from build123d import *

# Parameters (mm, degrees)
IZIM1_W                     = 12.4
IZIM1_H                     = 22.6
Y_KSEKLIK_EKSTR_ZYON1_DEPTH = 22.6
Y_KSEKLIK_EKSTR_ZYON2_DEPTH = 2.5
IZIM3_W                     = 3.6
IZIM3_H                     = 3
Y_KSEKLIK_EKSTR_ZYON3_DEPTH = 1.2
IZIM4_R                     = 6.2
Y_KSEKLIK_EKSTR_ZYON4_DEPTH = 4.25
IZIM5_R                     = 2.45
IZIM5_R_2                   = 0.6
Y_KSEKLIK_EKSTR_ZYON6_DEPTH = 3.15
IZIM6_W                     = 0.1
IZIM6_H                     = 1.2
KES_EKSTR_ZYON1_DEPTH       = 3
RADYUS1_R                   = 0.5


with BuildPart() as part:
    # Çizim1 → Yükseklik-Ekstrüzyon1 (new body)
    with BuildSketch(Plane(origin=(0, 0, 0), x_dir=(1, 0, 0), z_dir=(0, 1, 0))):
        Rectangle(IZIM1_W, IZIM1_H)
    extrude(amount=Y_KSEKLIK_EKSTR_ZYON1_DEPTH)

    # Çizim2 → Yükseklik-Ekstrüzyon2 (add)
    with BuildSketch(Plane(origin=(0, 18.2, 0), x_dir=(1, 0, 0), z_dir=(0, 1, 0))):
        with BuildLine():
            Line((-6.2, 16.125), (-6.2, -16.125))
            Line((-6.2, -16.125), (-0.5, -16.125))
            Line((-0.5, -16.125), (-0.5, -15.125))
            ThreePointArc((-0.5, -15.125), (-0.574456265, -13.207120951), (1.1, -14.145204103))
            ThreePointArc((1.1, -14.145204103), (0.938083152, -14.719660368), (0.5, -15.125))
            Line((0.5, -15.125), (0.5, -16.125))
            Line((0.5, -16.125), (6.2, -16.125))
            Line((6.2, -16.125), (6.2, 16.125))
            Line((6.2, 16.125), (0.5, 16.125))
            Line((0.5, 16.125), (0.5, 15.125))
            ThreePointArc((0.5, 15.125), (0.938083152, 14.719660368), (1.1, 14.145204103))
            ThreePointArc((1.1, 14.145204103), (-0.574456265, 13.207120951), (-0.5, 15.125))
            Line((-0.5, 15.125), (-0.5, 16.125))
            Line((-0.5, 16.125), (-6.2, 16.125))
        make_face()
    extrude(amount=-Y_KSEKLIK_EKSTR_ZYON2_DEPTH)

    # Çizim3 → Yükseklik-Ekstrüzyon3 (add)
    with BuildSketch(Plane(origin=(0, 4.8, 0), x_dir=(-1, 0, 0), z_dir=(0, -1, 0))):
        with Locations((0, 12.8)):
            Rectangle(IZIM3_W, IZIM3_H)
    extrude(amount=Y_KSEKLIK_EKSTR_ZYON3_DEPTH)

    # Çizim4 → Yükseklik-Ekstrüzyon4 (add)
    with BuildSketch(Plane(origin=(0, 22.6, 0), x_dir=(1, 0, 0), z_dir=(0, 1, 0))):
        with Locations((0, 5)):
            Circle(IZIM4_R)
        with BuildLine():
            Line((-2.7, -0.581218505), (-2.7, -0.7))
            ThreePointArc((-2.7, -0.7), (0, -3.4), (2.7, -0.7))
            Line((2.7, -0.7), (2.7, -0.581218505))
            ThreePointArc((2.7, -0.581218505), (0, -1.2), (-2.7, -0.581218505))
        make_face()
    extrude(amount=Y_KSEKLIK_EKSTR_ZYON4_DEPTH)

    # Çizim5 → Yükseklik-Ekstrüzyon6 (add)
    with BuildSketch(Plane(origin=(0, 26.85, 0), x_dir=(1, 0, 0), z_dir=(0, 1, 0))):
        with Locations((0, 5)):
            Circle(IZIM5_R)
        with Locations((0, 5)):
            Circle(IZIM5_R_2, mode=Mode.SUBTRACT)
    extrude(amount=Y_KSEKLIK_EKSTR_ZYON6_DEPTH)

    # Çizim6 → Kes-Ekstrüzyon1 (cut)
    with BuildSketch(Plane(origin=(0, 0, -14.3), x_dir=(-1, 0, 0), z_dir=(0, 0, -1))):
        with Locations((-0.616666667, 4.2)):
            Rectangle(IZIM6_W, IZIM6_H)
        with Locations((0.616666667, 4.2)):
            Rectangle(IZIM6_W, IZIM6_H)
    extrude(amount=-KES_EKSTR_ZYON1_DEPTH, mode=Mode.SUBTRACT)

    # Radyus1
    radyus1_edges = [part.edges().sort_by_distance(p)[0] for p in [
        (0.566666667, 3.6, -12.8),
        (0.566666667, 4.8, -12.8),
        (0.666666667, 4.8, -12.8),
        (0.666666667, 3.6, -12.8),
        (-0.666666667, 3.6, -12.8),
        (-0.666666667, 4.8, -12.8),
        (-0.566666667, 4.8, -12.8),
        (-0.566666667, 3.6, -12.8),
        (1.8, 4.8, -12.8),
        (-1.8, 4.8, -12.8),
        (1.8, 3.6, -12.8),
        (-1.8, 3.6, -12.8),
    ]]
    fillet(radyus1_edges, radius=RADYUS1_R)


solid = part.part
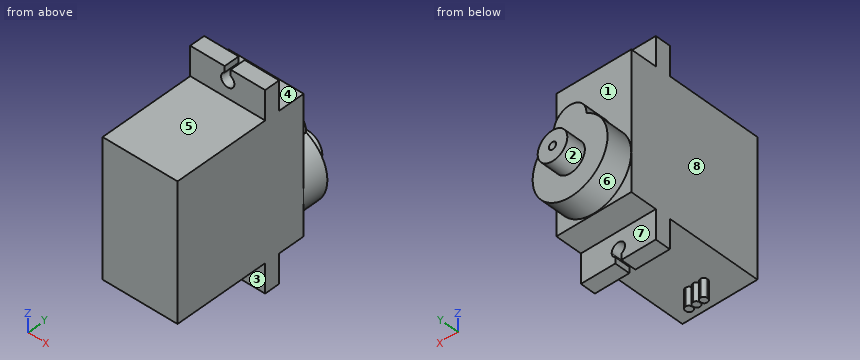
Build history of the part. All positions in model axes, mm. Face numbers are marked on the shaded views. A direction names the side the tool comes from. Coordinates: 2 decimals unless noted, no trailing zeros. Write each loop counter-clockwise with the first axis right and the second up, starting at its lowest first coordinate (ties: lowest second). Pieces come first, ordered by that corner, then holes. Notation, with made-up numbers: (-14, -4) -> (11, -4) arc R30 cw to (11, 34) -> close; hole circle Ø5 at (32, -4.75). An arc over 180 degrees is marked (long way). Use CSV: the item, a comma, the result in double quotes. Start each with the question number.
Q1. Cut at A-A, the plane z = 2.5. List the corners of the cut face in (x, y).
Q2. Cut at C-C, the plane y = 13.75. List the corners of the cut face in (x, z), then the cut area to 3 significant figures.
Q3. Cut at B-B, the plane x = -5. List the corners of the cut face in (y, z) (3 decimals).
Q4. Drill centre lines: probe 1 along Y at (x, z) = (0, -12); probe 2 along Z at (x, y) = (0, 17.25); probe 3 along Z at (x, y) = (5, 10.5). Where is each one in solid material? Low to high.
Q5. Pull direction Y, two halves, no side cores. Call the marked faces 1, 2 and 3: released by +Y, released by -Y, zero draft, split by the parting line, or undercut.
Q6. Flat gauge pins, fed straight in: pin 1 Ø2 at (x, y) = (0, 20.5) entering from -Z; pin 2 Ø1.5 at (x, y) = (4, 5) entering from +Z; pin 3 Ø1.8 at (x, z) = (0, -14.15) entering from +Y. Where does each tip first touch, or does it go through?
Q7. 3-axis set-ups, long thin cutter, end or side, ignore diameter. For the marked faces 4, 5, 6, 7 and 8: which of +Z, -Z, +X, -X, +Y, -Y reach the whole face in a straight line?
Q8. Cut at D-D, the plane y = 26. List the corners of the cut face in (x, z).
Checked values:
1,outline,"(-6.2, 0) -> (6.2, 0) -> (6.2, 22.6) -> (2.01, 22.6) -> (2.01, 26.85) -> (-2.01, 26.85) -> (-2.01, 22.6) -> (-6.2, 22.6) -> close"
2,outline,"(-6.2, -11.3) -> (6.2, -11.3) -> (6.2, 11.3) -> (-6.2, 11.3) -> close"
2,area,"280 mm²"
3,outline,"(0, -11.3) -> (15.7, -11.3) -> (15.7, -16.125) -> (18.2, -16.125) -> (18.2, -11.3) -> (22.6, -11.3) -> (22.6, -8.666) -> (26.85, -8.666) -> (26.85, -1.334) -> (22.6, -1.334) -> (22.6, 11.3) -> (18.2, 11.3) -> (18.2, 16.125) -> (15.7, 16.125) -> (15.7, 11.3) -> (0, 11.3) -> close"
4,probe 1,"y = 3.6 to 4.8, 15.7 to 18.2"
4,probe 2,"z = -13.05 to 13.05"
4,probe 3,"z = -11.3 to 11.3"
5,face 1,"released by +Y"
5,face 2,"zero draft"
5,face 3,"undercut"
6,pin 1,"stops at z = -11.3"
6,pin 2,"stops at z = 11.3"
6,pin 3,"stops at y = 4.8"
7,face 4,"+Z, +X, -X, +Y"
7,face 5,"+Z, +X, -X, -Y"
7,face 6,"+Y"
7,face 7,"-Z, +X, -X, +Y"
7,face 8,"+Z, -Z, -X, +Y, -Y"
8,outline,"(-2.7, 0.58) arc R6.2 ccw (long way) to (2.7, 0.58) -> (2.7, 0.7) arc R2.7 ccw to (-2.7, 0.7) -> close"
